Part model, mm, in its own coordinate system. A direction names the side the tool comes from. Round coordinates to 2 decimals unless told otherwise and drop trailing zeros. Write each loop counter-clockwise with the first axis right and the second up, starting at its lowest first coordinate (ties: lowest second). Pieces come first, ordered by that corner, then holes. Notation, with made-up numbers: M 48,20 L 90,20 A14 ccw 90,42 Z; hole C -18.75,88.25 d1. An arc over 180 degrees is marked long. Use one line per item in the form item = value. Start each with the question number.
Item 1: Flat gauge pins, fed straight in: pin 1 Ø2 at (x, z) = (12, 8) entering from +Y; pin 2 Ø1 at (x, z) = (19.5, 4) entering from +Y; pin 3 Ø4 at (y, z) = (4, 3) entering from +X; pin 4 Ø1 at (x, z) = (32, 3) entering from +Y. Where does each tip first touch, or does it go through?
Item 2: Cut at A-A, the plane z = 4.75. Give the cut face in (x, y).
Item 3: Probe L1, parallel to Z at x = 21, y = -1.5; L2, parallel to X at y = 1, z = 9; L3, parallel to X at y = -3.25, z = 4.25. List the from-to ranges inside material, lowest first.
Item 4: Mould opens along X. For faces 3 (the face through (23, 0, 0)), 4 (the face through (16.869, -0.436, 9.076)), 5 (the face through (10.691, 2.935, 0.246)) say: +X half, -X half, draft (parallel to the pull), parting line (faces both ways), or undercut.
Item 5: Cut at D-D, the plane y = 6.25. Give the cut face in (x, z).
Item 6: Cut at C-C, the plane z = 8.75. Give the cut face in (x, y), then the cut area to 3 significant figures.
Item 7: Cut at B-B, the plane y = -4.5. Give the cut face in (x, z), then the cut area to 3 significant figures.
Item 8: Which spindle directions (+Z, -Z, +X, -X, +Y, -Y) get a long thin tool onto all of the face, cutting with end or side? Do faces 1 (the face through (8.724, 0.601, 2.965)), 2 (the face through (3.498, -1.467, 0.246)). Say none if no direction does.
from build123d import *

# Parameters (mm, degrees)
F1_DEPTH = 0.5
F2_R     = 2
F2_R_2   = 1
F2_R_3   = 4
F2_R_4   = 8
F3_DEPTH = 10
F4_SIZE2 = 5
F4_SIZE  = 1
F5_R     = 8
F6_SIZE2 = 5
F6_SIZE  = 2
F7_SIZE2 = 5
F7_SIZE  = 4


with BuildPart() as f1:
    # F0 (on Top) → F1 (new body)
    with BuildSketch(Plane.XY):
        with BuildLine():
            ThreePointArc((28.6830315128, -7.7103105572), (35.6606054127, -6.366579406), (38.8163648461, 0))
            ThreePointArc((38.8163648461, 0), (35.6606054127, 6.366579406), (28.6830315128, 7.7103105572))
            ThreePointArc((28.6830315128, 7.7103105572), (22.8163648461, 0), (28.6830315128, -7.7103105572))
        make_face()
        with BuildLine():
            ThreePointArc((28.6830315128, -7.7103105572), (22.8163648461, 0), (28.6830315128, 7.7103105572))
            Line((28.6830315128, 7.7103105572), (14.8380732426, 3.8796074024))
            Line((14.8380732426, 3.8796074024), (6.4271638375, 1.9625832337))
            Line((6.4271638375, 1.9625832337), (0.6496981795, 0.9860132972))
            ThreePointArc((0.6496981795, 0.9860132972), (1.4618620705, 0.7637626158), (1.8163648461, 0))
            ThreePointArc((1.8163648461, 0), (1.4618620705, -0.7637626158), (0.6496981795, -0.9860132972))
            Line((0.6496981795, -0.9860132972), (6.4271638375, -1.9625832337))
            Line((6.4271638375, -1.9625832337), (14.8380732426, -3.8796074024))
            Line((14.8380732426, -3.8796074024), (28.6830315128, -7.7103105572))
        make_face()
        with BuildLine():
            ThreePointArc((1.8163648461, 0), (1.4618620705, 0.7637626158), (0.6496981795, 0.9860132972))
            ThreePointArc((0.6496981795, 0.9860132972), (-0.1836351539, 0), (0.6496981795, -0.9860132972))
            ThreePointArc((0.6496981795, -0.9860132972), (1.4618620705, -0.7637626158), (1.8163648461, 0))
        make_face()
    extrude(amount=F1_DEPTH)

    # F2 (on face) → F3 (join)
    with BuildSketch(Plane.XY.offset(0.5)):
        with Locations((6.8163648461, 0)):
            Circle(F2_R)
        with Locations((0.8163648461, 0)):
            Circle(F2_R_2)
        with Locations((15.8163648461, 0)):
            Circle(F2_R_3)
        with Locations((30.8163648461, 0)):
            Circle(F2_R_4)
    extrude(amount=F3_DEPTH)

    # F4
    f4_edges = [f1.edges().sort_by_distance(p)[0] for p in [
        (-0.183635, 0, 10.5),
    ]]
    f4_side = f1.faces().sort_by_distance((0.816365, 0, 10.5))[0]
    chamfer(f4_edges, length=F4_SIZE, length2=F4_SIZE2, reference=f4_side)

    # F5
    f5_edges = [f1.edges().sort_by_distance(p)[0] for p in [
        (22.816365, 0, 10.5),
    ]]
    fillet(f5_edges, radius=F5_R)

    # F6
    f6_edges = [f1.edges().sort_by_distance(p)[0] for p in [
        (4.816365, 0, 10.5),
    ]]
    f6_side = f1.faces().sort_by_distance((6.816365, 0, 10.5))[0]
    chamfer(f6_edges, length=F6_SIZE, length2=F6_SIZE2, reference=f6_side)

    # F7
    f7_edges = [f1.edges().sort_by_distance(p)[0] for p in [
        (11.816365, 0, 10.5),
    ]]
    f7_side = f1.faces().sort_by_distance((15.816365, 0, 10.5))[0]
    chamfer(f7_edges, length=F7_SIZE, length2=F7_SIZE2, reference=f7_side)


solid = f1.part
Model answer:
q1.pin_1 = through
q1.pin_2 = 2.42
q1.pin_3 = 38.55
q1.pin_4 = 7.96
q2.outline = C 0.82,0 d2; C 6.82,0 d4; C 15.82,0 d8; C 30.82,0 d15.35
q3.L1 = 0 to 0.5
q3.L2 = 15.15 to 16.48, 26.26 to 35.37
q3.L3 = 13.48 to 18.15, 23.72 to 37.91
q4.face_3 = draft
q4.face_4 = undercut
q4.face_5 = -X half
q5.outline = M 23.41,0 L 35.81,0 L 35.81,2.5 A4.99 ccw 25.82,2.5 L 25.82,0.5 L 23.41,0.5 Z
q6.outline = C 0.82,0 d0.7; C 6.82,0 d1.4; C 15.82,0 d2.8; C 30.82,0 d9.99
q6.area = 86.4 mm²
q7.outline = M 17.08,0 L 37.43,0 L 37.43,2.5 A6.61 ccw 24.2,2.5 L 24.2,0.5 L 17.08,0.5 Z
q7.area = 105 mm²
q8.face_1 = +Z
q8.face_2 = +Z, -Z, -X, -Y
